from build123d import *

# Parameters (mm, degrees)
SKETCH_1_W      = 30
SKETCH_1_H      = 10
EXTRUDE_1_DEPTH = 16.2
SKETCH_2_R      = 0.45
EXTRUDE_2_DEPTH = 4


with BuildPart() as part:
    # Эскиз1 → Бобышка-Вытянуть1 (new body)
    with BuildSketch(Plane.XY):
        Rectangle(SKETCH_1_W, SKETCH_1_H)
    extrude(amount=EXTRUDE_1_DEPTH)

    # Эскиз2 → Бобышка-Вытянуть2 (add)
    with BuildSketch(Plane(origin=(0, 0, 0), x_dir=(-1, 0, 0), z_dir=(0, 0, -1))):
        with Locations((-13.5, 3.8)):
            Circle(SKETCH_2_R)
        with Locations((-7.1, 3.8)):
            Circle(SKETCH_2_R)
        with Locations((-10.3, -3.8)):
            Circle(SKETCH_2_R)
        with Locations((11.9, 3.8)):
            Circle(SKETCH_2_R)
        with Locations((11.9, -3.8)):
            Circle(SKETCH_2_R)
    extrude(amount=EXTRUDE_2_DEPTH)


solid = part.part
Source: CAD feature listing. Evaluate the final solid. Frame: model axes, mm. A direction names the side the tool comes from. Round coordinates to 2 decimals unless told otherwise and drop trailing zeros. Loops run counter-clockwise (first coordinate to the right, second up) from the corner with the lowest first, then second, coordinate; pieces in that order, holes last.
Q1. Section B-B, the plane y = -3.8. Return loops of the section in (x, z), plus the area to 3 significant figures.
Q2. Section C-C, the plane x = 10.3. Return loops of the section in (y, z).
Q3. Ray query, line 1 (Z direction, x = -10.75, y = 4). Return the intervals inside material, ascending.
Q4. Mould query, pull axis X, two halves, no side actions, for faces 1 (the face through (10.3, -3.8, -4)), 2 (the face through (9.884, -3.972, -1.972)), 3 (the face through (-15, 0, 8)), 4 (the face through (15, 0, 8)). Classes: pulls with the +X half, pulls with the -X half, needs draft (parallel to the pull), parting line crosses it, or undercut.
Q5. Access query for faces 5 (the face through (-12, -4, -4)), 6 (the face through (7.159, 4.246, -1.972)). Directions: +Z, -Z, +X, -X, +Y, -Y. A direction counts if a zero-diameter tool reaches every point of the face in a straight line with its end or side. Return the directions, or none.
Q6. Section D-D, the plane x = -11.9. Return loops of the section in (y, z).
Q7. Section A-A, the plane z = -1.75. Return loops of the section in (x, y).
Solutions:
1. outline: (-15, 0) - (-12.35, 0) - (-12.35, -4) - (-11.45, -4) - (-11.45, 0) - (9.85, 0) - (9.85, -4) - (10.75, -4) - (10.75, 0) - (15, 0) - (15, 16.2) - (-15, 16.2) - close
1. area: 493 mm2
2. outline: (-5, 0) - (-4.25, 0) - (-4.25, -4) - (-3.35, -4) - (-3.35, 0) - (5, 0) - (5, 16.2) - (-5, 16.2) - close
3. line 1: z = 0 to 16.2
4. face 1: needs draft
4. face 2: undercut
4. face 3: pulls with the -X half
4. face 4: pulls with the +X half
5. face 5: -Z, +X, -X, +Y, -Y
5. face 6: -Z
6. outline: (-5, 0) - (-4.25, 0) - (-4.25, -4) - (-3.35, -4) - (-3.35, 0) - (3.35, 0) - (3.35, -4) - (4.25, -4) - (4.25, 0) - (5, 0) - (5, 16.2) - (-5, 16.2) - close
7. outline: circle Ø0.9 at (-11.9, -3.8); circle Ø0.9 at (-11.9, 3.8); circle Ø0.9 at (7.1, 3.8); circle Ø0.9 at (10.3, -3.8); circle Ø0.9 at (13.5, 3.8)
